Verification items for the finished model (mm, model axes). Face numbers are marked on the shaded views. A direction names the side the tool comes from. Give positions to 0.01 mm unless a question says otherwise; leave off trailing zeros. Loops run counter-clockwise (first coordinate to the right, second up) from the corner with the lowest first, then second, coordinate; pieces in that order, holes last. Notation, with made-up numbers: (-26.5, 36) - (-4.5, 36) arc R16 cw to (-4.5, 59) - close; hole circle Ø3 at (73, 88). An arc over 180 degrees is marked (long way). Use one line per item in the form item = value.
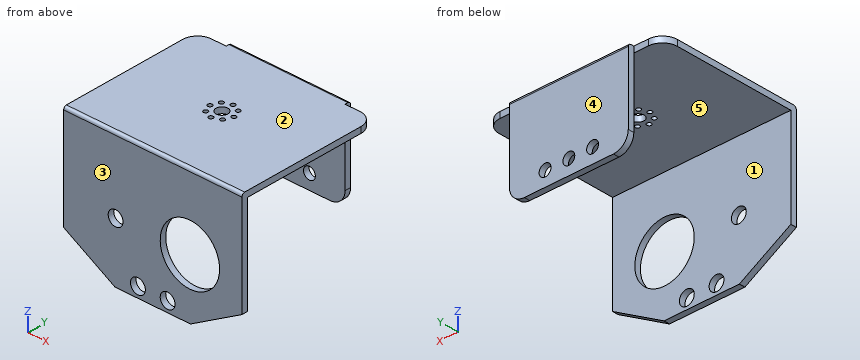
```python
from build123d import *

# Parameters (mm, degrees)
EXTRUDE_1_DEPTH     = 2
EXTRUDE_START       = -2
SKETCH_2_W          = 60
SKETCH_2_H          = 2
EXTRUDE_2_DEPTH     = 50
FILLET_1_R          = 1
SKETCH_3_W          = 20
SKETCH_3_H          = 2
EXTRUDE_4_DEPTH     = 30
SKETCH_3_3_W        = 10
SKETCH_3_3_H        = 2
CUT_EXTRUDE_1_DEPTH = 30
FILLET_4_R          = 5
FILLET_5_R          = 1
SKETCH_4_R          = 2
CUT_EXTRUDE_2_DEPTH = 30
FILLET_6_R          = 5
SKETCH_5_R          = 2.5
SKETCH_5_R_2        = 10
CUT_EXTRUDE_4_DEPTH = 30
SKETCH_6_R          = 2.5
CUT_EXTRUDE_5_DEPTH = 10
SKETCH_7_R          = 2
SKETCH_7_R_2        = 0.75
CUT_EXTRUDE_6_DEPTH = 10


with BuildPart() as part:
    # 草图1 → 凸台-拉伸1 (new body)
    with BuildSketch(Plane(origin=(0, 0, 0), x_dir=(1, 0, 0), z_dir=(0, 1, 0))):
        Polygon((-12.679491924, 0), (12.679491924, 0), (30, -10), (30, -45), (-30, -45), (-30, -10), align=None)
    extrude(amount=EXTRUDE_1_DEPTH)

    # 草图2 → 凸台-拉伸2 (add)
    with BuildSketch(Plane(origin=(0, 2, 0), x_dir=(1, 0, 0), z_dir=(0, 1, 0)).offset(EXTRUDE_START)):
        with Locations((0, -44)):
            Rectangle(SKETCH_2_W, SKETCH_2_H)
    extrude(amount=EXTRUDE_2_DEPTH)

    # 圆角1
    fillet_1_edges = [part.edges().sort_by_distance(p)[0] for p in [
        (0, 0, 45),
    ]]
    fillet(fillet_1_edges, radius=FILLET_1_R)

    # 草图3 → 凸台-拉伸4 (add)
    with BuildSketch(Plane(origin=(0, 0, 43), x_dir=(-1, 0, 0), z_dir=(0, 0, -1)).offset(EXTRUDE_START)):
        with Locations((-10, 49)):
            Rectangle(SKETCH_3_W, SKETCH_3_H)
        with Locations((10, 49)):
            Rectangle(SKETCH_3_W, SKETCH_3_H)
    extrude(amount=EXTRUDE_4_DEPTH)

    # 草图3<3> → 切除-拉伸1 (cut)
    with BuildSketch(Plane(origin=(0, 0, 43), x_dir=(-1, 0, 0), z_dir=(0, 0, -1))):
        with Locations((-25, 49)):
            Rectangle(SKETCH_3_3_W, SKETCH_3_3_H)
        with Locations((25, 49)):
            Rectangle(SKETCH_3_3_W, SKETCH_3_3_H)
    extrude(amount=-CUT_EXTRUDE_1_DEPTH, mode=Mode.SUBTRACT)

    # 圆角4
    fillet_4_edges = [part.edges().sort_by_distance(p)[0] for p in [
        (30, 48, 44),
        (-30, 48, 44),
    ]]
    fillet(fillet_4_edges, radius=FILLET_4_R)

    # 圆角5
    fillet_5_edges = [part.edges().sort_by_distance(p)[0] for p in [
        (0, 50, 45),
    ]]
    fillet(fillet_5_edges, radius=FILLET_5_R)

    # 草图4 → 切除-拉伸2 (cut)
    with BuildSketch(Plane(origin=(0, 50, 0), x_dir=(1, 0, 0), z_dir=(0, 1, 0))):
        with Locations(Location((0, -20, 0), (0, 0, 270))):
            Circle(SKETCH_4_R)
        with Locations(Location((-8, -20, 0), (0, 0, 270))):
            Circle(SKETCH_4_R)
        with Locations(Location((8, -20, 0), (0, 0, 270))):
            Circle(SKETCH_4_R)
    extrude(amount=-CUT_EXTRUDE_2_DEPTH, mode=Mode.SUBTRACT)

    # 圆角6
    fillet_6_edges = [part.edges().sort_by_distance(p)[0] for p in [
        (-20, 49, 15),
        (20, 49, 15),
    ]]
    fillet(fillet_6_edges, radius=FILLET_6_R)

    # 草图5 → 切除-拉伸4 (cut)
    with BuildSketch(Plane.XZ):
        with Locations(Location((-12.5, 20, 0), (0, 0, 270))):
            Circle(SKETCH_5_R)
        with Locations(Location((12.5, 20, 0), (0, 0, 270))):
            Circle(SKETCH_5_R_2)
    extrude(amount=-CUT_EXTRUDE_4_DEPTH, mode=Mode.SUBTRACT)

    # 草图6 → 切除-拉伸5 (cut)
    with BuildSketch(Plane(origin=(0, 2, 0), x_dir=(1, 0, 0), z_dir=(0, 1, 0))):
        with Locations(Location((5, -3.5, 0), (0, 0, 270))):
            Circle(SKETCH_6_R)
        with Locations(Location((-5, -3.5, 0), (0, 0, 270))):
            Circle(SKETCH_6_R)
    extrude(amount=-CUT_EXTRUDE_5_DEPTH, mode=Mode.SUBTRACT)

    # 草图7 → 切除-拉伸6 (cut)
    with BuildSketch(Plane.XY.offset(45)):
        with Locations((0, 25)):
            Circle(SKETCH_7_R)
        with Locations((0, 29)):
            Circle(SKETCH_7_R_2)
        with Locations((2.828427125, 27.828427125)):
            Circle(SKETCH_7_R_2)
        with Locations((4, 25)):
            Circle(SKETCH_7_R_2)
        with Locations((2.828427125, 22.171572875)):
            Circle(SKETCH_7_R_2)
        with Locations((0, 21)):
            Circle(SKETCH_7_R_2)
        with Locations((-2.828427125, 22.171572875)):
            Circle(SKETCH_7_R_2)
        with Locations((-4, 25)):
            Circle(SKETCH_7_R_2)
        with Locations((-2.828427125, 27.828427125)):
            Circle(SKETCH_7_R_2)
    extrude(amount=-CUT_EXTRUDE_6_DEPTH, mode=Mode.SUBTRACT)


solid = part.part
```
1. Section check C-C, the plane z = 12.5. Record the cut outline in (x, y), then the cut area to 3 significant figures.
Result set:
outline = (-30, 0) - (5.89, 0) - (5.89, 2) - (-30, 2) - close; (19.11, 0) - (30, 0) - (30, 2) - (19.11, 2) - close
area = 93.5 mm²
2. Tool access check on the marked faces 1 and 2. Record the directions out of +Z, -Z, +X, -X, +Y, -Y that give a thin tool (end or side, any length) a straight path to the whole face; none if there is none.
Result set:
face_1 = -Z, +X, -X
face_2 = +Z, +X, -X, +Y, -Y
3. Depth check by flat-ended pin: pin 1 Ø2 at (x, y) = (0, 21) entering from -Z; pin 2 Ø5 at (y, z) = (10.5, 39) entering from -X; pin 3 Ø6 at (x, z) = (10, 26.5) entering from -Y; pin 4 Ø8 at (x, z) = (5, 3.5) entering from +Y. Enter the tip coordinate at first touch or a pass-through.
Result set:
pin_1 = 43
pin_2 = through
pin_3 = 48
pin_4 = 2
4. Section check B-B, the plane x = -16. Record the cut outline in (y, z).
Result set:
outline = (0, 1.92) - (2, 1.92) - (2, 43) - (48, 43) - (48, 15.1) - (50, 15.1) - (50, 44) arc R1 ccw to (49, 45) - (1, 45) arc R1 ccw to (0, 44) - close
5. Scan lines: probe 1 along X at (y, z) = (48.55, 20); probe 2 along Y at (x, z) = (-12.5, 35.5); probe 3 along X at (y, z) = (0.85, 20). Record each from-to range of solid material in increasing order.
Result set:
probe_1 = -20 to -10, -6 to -2, 2 to 6, 10 to 20
probe_2 = 0 to 2, 48 to 50
probe_3 = -30 to -15, -10 to 2.5, 22.5 to 30
6. Section check D-D, the plane y = 10. Record the cut outline in (x, z), then the cut area to 3 significant figures.
Result set:
outline = (-30, 43) - (30, 43) - (30, 45) - (-30, 45) - close
area = 120 mm²
7. Section check A-A, the plane z = 28. Record the cut outline in (x, y), then the cut area to 3 significant figures.
Result set:
outline = (-30, 0) - (6.5, 0) - (6.5, 2) - (-30, 2) - close; (-20, 48) - (20, 48) - (20, 50) - (-20, 50) - close; (18.5, 0) - (30, 0) - (30, 2) - (18.5, 2) - close
area = 176 mm²
8. Draft check along Y on the marked faces 3, 4 and 5. Enter one of: released by +Y, released by -Y, zero draft, split by the parting line, or undercut.
Result set:
face_3 = released by -Y
face_4 = released by +Y
face_5 = undercut
